from build123d import *

# Parameters (mm, degrees)
SKETCH1_R           = 2
BOSS_EXTRUDE1_DEPTH = 5
BOSS_EXTRUDE2_DEPTH = 20
FILLET1_R           = 5


with BuildPart() as part:
    # Sketch1 → Boss-Extrude1 (new body)
    with BuildSketch(Plane.XY):
        with BuildLine():
            ThreePointArc((19.213203177, 21.000000313), (-29.5, 3.499999932), (19.213203263, -14.000000209))
            Line((19.213203263, -14.000000209), (43.5, -14.000000209))
            Line((43.5, -14.000000209), (43.5, -40))
            ThreePointArc((43.5, -40), (39.985281374, -48.485281374), (31.5, -52))
            Line((31.5, -52), (-43.5, -52))
            Line((-43.5, -52), (-43.5, 52))
            Line((-43.5, 52), (31.5, 52))
            ThreePointArc((31.5, 52), (39.985281374, 48.485281374), (43.5, 40))
            Line((43.5, 40), (43.5, 21.000000313))
            Line((43.5, 21.000000313), (19.213203177, 21.000000313))
        make_face()
        with Locations((9.5, 42)):
            Circle(SKETCH1_R, mode=Mode.SUBTRACT)
        with Locations((-21.5, -42)):
            Circle(SKETCH1_R, mode=Mode.SUBTRACT)
        with Locations((9.5, -42)):
            Circle(SKETCH1_R, mode=Mode.SUBTRACT)
        with Locations((-21.5, 42)):
            Circle(SKETCH1_R, mode=Mode.SUBTRACT)
    extrude(amount=BOSS_EXTRUDE1_DEPTH)

    # Sketch1_3 → Boss-Extrude2 (add)
    with BuildSketch(Plane.XY):
        with BuildLine():
            ThreePointArc((16.582585934, 6), (-20.75, 3.5), (16.582585934, 1))
            Line((16.582585934, 1), (39.5, 1))
            Line((39.5, 1), (43.5, 1))
            Line((43.5, 1), (43.5, -14.000000209))
            Line((43.5, -14.000000209), (19.213203263, -14.000000209))
            ThreePointArc((19.213203263, -14.000000209), (-29.5, 3.499999932), (19.213203177, 21.000000313))
            Line((19.213203177, 21.000000313), (43.5, 21.000000313))
            Line((43.5, 21.000000313), (43.5, 6))
            Line((43.5, 6), (39.5, 6))
            Line((39.5, 6), (16.582585934, 6))
        make_face()
    extrude(amount=BOSS_EXTRUDE2_DEPTH)

    # Fillet1
    fillet1_edges = [part.edges().sort_by_distance(p)[0] for p in [
        (43.5, 13.500000156, 20),
        (43.5, -6.500000104, 20),
    ]]
    fillet(fillet1_edges, radius=FILLET1_R)


solid = part.part
Model file for the job. Use its own axes, mm. A direction names the side the tool comes from. Coordinates: 2 decimals unless noted, no trailing zeros. Write each loop counter-clockwise with the first axis right and the second up, starting at its lowest first coordinate (ties: lowest second). Pieces come first, ordered by that corner, then holes. Notation, with made-up numbers: (45, 88.25) -> (87, 88.25) arc R22 cw to (87, 98.25) -> close; hole circle Ø10 at (37.5, 5). An arc over 180 degrees is marked (long way). One line per item, written item: value. Start each with the question number.
1) Which spindle directions (+Z, -Z, +X, -X, +Y, -Y) get a long thin tool onto all of the face, cutting with end or side? Do faces 4 (the face through (-29.484, 2.556, 12.395)), 5 (the face through (30, 6, 10)), 6 (the face through (31, 21, 12)). Say none if no direction does.
2) Slice it at A-A on x = -2. Write the cut outline in (y, z).
3) Slice it at C-C on x = 9.5. Write the cut outline in (y, z), then the cut area to 3 significant figures.
4) Probe probe 1 along Y at (x, z) = (-21.5, 3.5); probe 2 along Y at (x, z) = (29.5, 6.5); probe 3 along Y at (x, z) = (9.5, 1.3). List the from-to ranges inside material, lowest first.
5) Slice it at B-B on y = 17.5. Write the cut outline in (x, z).
6) Flat gauge pins, fed straight in: pin 1 Ø5 at (x, y) = (9.5, -42) entering from +Z; pin 2 Ø4.5 at (x, z) = (30, 10) entering from -Y; pin 3 Ø7.5 at (x, z) = (25.5, 14.5) entering from +Y. Where does each tip first touch, or does it go through?
7) Pull direction X, two halves, no side cores. Call faces 1 (the face through (9.066, 40.048, 2.465)), 2 (the face through (40.08, -48.39, 2.46)), 3 (the face through (-7, 52, 2)): +X half, -X half, draft (parallel to the pull), parting line (faces both ways), or undercut.
8) Slice it at D-D on z = 8.75. Write the cut outline in (x, y), then the cut area to 3 significant figures.
Answers follow:
1. face 4: +Z
1. face 5: +Z, -Z, +X
1. face 6: +Z, +X, +Y
2. outline: (-52, 0) -> (-15.25, 0) -> (-15.25, 20) -> (-24, 20) -> (-24, 5) -> (-52, 5) -> close; (22.25, 0) -> (52, 0) -> (52, 5) -> (31, 5) -> (31, 20) -> (22.25, 20) -> close
3. outline: (-52, 0) -> (-44, 0) -> (-44, 5) -> (-52, 5) -> close; (-40, 0) -> (-11.31, 0) -> (-11.31, 20) -> (-21.48, 20) -> (-21.48, 5) -> (-40, 5) -> close; (18.31, 0) -> (40, 0) -> (40, 5) -> (28.48, 5) -> (28.48, 20) -> (18.31, 20) -> close; (44, 0) -> (52, 0) -> (52, 5) -> (44, 5) -> close
3. area: 637 mm2
4. probe 1: -52 to -44, -40 to 40, 44 to 52
4. probe 2: -14 to 1, 6 to 21
4. probe 3: -52 to -44, -40 to -11.31, 18.31 to 40, 44 to 52
5. outline: (-43.5, 0) -> (-14.47, 0) -> (-14.47, 20) -> (-25.67, 20) -> (-25.67, 5) -> (-43.5, 5) -> close; (10.47, 0) -> (43.5, 0) -> (43.5, 15) arc R5 ccw to (38.5, 20) -> (10.47, 20) -> close
6. pin 1: z = 5
6. pin 2: y = -14
6. pin 3: y = 21
7. face 1: undercut
7. face 2: +X half
7. face 3: draft
8. outline: (16.58, 1) arc R18.75 cw (long way) to (16.58, 6) -> (43.5, 6) -> (43.5, 21) -> (19.21, 21) arc R27.5 ccw (long way) to (19.21, -14) -> (43.5, -14) -> (43.5, 1) -> close
8. area: 1,840 mm2
